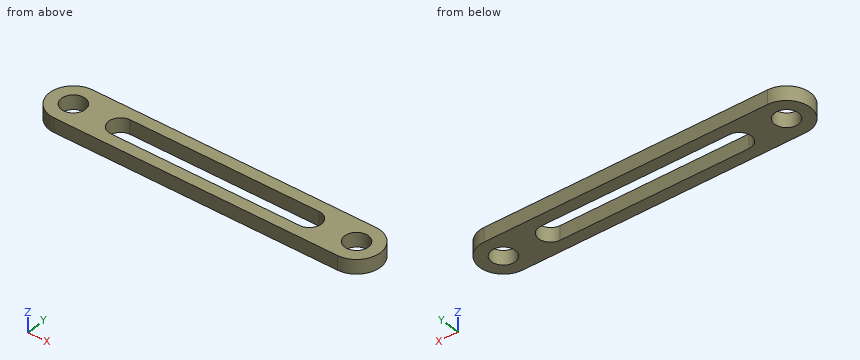
from build123d import *

# Parameters (mm, degrees)
F0_R     = 2.5
F1_DEPTH = 3


with BuildPart() as f1:
    # F0 (on Top) → F1 (new body)
    with BuildSketch(Plane.XY):
        with BuildLine():
            Line((60, 5), (0, 5))
            ThreePointArc((0, 5), (-5, 0), (0, -5))
            Line((0, -5), (60, -5))
            ThreePointArc((60, -5), (65, 0), (60, 5))
        make_face()
        Circle(F0_R, mode=Mode.SUBTRACT)
        with BuildLine():
            ThreePointArc((10, -2.5), (7.5, 0), (10, 2.5))
            Line((10, 2.5), (50, 2.5))
            ThreePointArc((50, 2.5), (52.5, 0), (50, -2.5))
            Line((50, -2.5), (10, -2.5))
        make_face(mode=Mode.SUBTRACT)
        with Locations((60, 0)):
            Circle(F0_R, mode=Mode.SUBTRACT)
    extrude(amount=F1_DEPTH)


solid = f1.part
Check sheet for the modelled part. Datum: model origin and axes. Units: mm. Round coordinates to 2 decimals unless told otherwise and drop trailing zeros. Loops run counter-clockwise (first coordinate to the right, second up) from the corner with the lowest first, then second, coordinate; pieces in that order, holes last. Notation, with made-up numbers: M 75.25,47.5 L 97.25,47.5 A4 cw 97.25,53.5 Z; hole C 12,30.25 d1. An arc over 180 degrees is marked long. One line per item, written item: value.
(1) Sectioned sample at B-B, the plane x = 9. Record the cut outline in (y, z), then the cut area to 3 significant figures.
Computed values:
outline: M -5,0 L -2.29,0 L -2.29,3 L -5,3 Z; M 2.29,0 L 5,0 L 5,3 L 2.29,3 Z
area: 16.3 mm^2
(2) Sectioned sample at C-C, the plane x = 43.5. Record the cut outline in (y, z), then the cut area to 3 significant figures.
Computed values:
outline: M -5,0 L -2.5,0 L -2.5,3 L -5,3 Z; M 2.5,0 L 5,0 L 5,3 L 2.5,3 Z
area: 15.0 mm^2
(3) Thickness scan on line 1 (Y direction, x = 21.5, z = 1.5); line 2 (X direction, y = 2, z = 2.35); line 3 (X direction, y = -1.75, z = 1). Record the ranges inside material, lowest first.
Computed values:
line 1: y = -5 to -2.5, 2.5 to 5
line 2: x = -4.58 to -1.5, 1.5 to 8.5, 51.5 to 58.5, 61.5 to 64.58
line 3: x = -4.68 to -1.79, 1.79 to 8.21, 51.79 to 58.21, 61.79 to 64.68
(4) Sectioned sample at A-A, the plane z = 0.95. Record the cut outline in (x, y).
Computed values:
outline: M 0,-5 L 60,-5 A5 ccw 60,5 L 0,5 A5 ccw Z; hole C 0,0 d5; hole M 10,-2.5 L 50,-2.5 A2.5 ccw 50,2.5 L 10,2.5 A2.5 ccw Z; hole C 60,0 d5
